Autodesk Fusion 360 part; units mm, degrees
sketch "Boceto1" plane through (0, 0, 0) normal (0, 0, 1) x (1, 0, 0)
  line L0 (0, -31.5) -> (3, -31.5) construction
  circle A0 centre (3, -22.5) radius 1.5 construction
  circle A1 centre (3, -10.5) radius 1.5 construction
  circle A2 centre (-5.5, -17.5) radius 1.5 construction
  line L1 (0, -35) -> (0, -31.5) construction
  line L2 (0, -35) -> (0, -5) construction
  line L3 (0, -20) -> (7.4517, -20) construction
  circle A3 centre (0, -16.5) radius 1.5 construction
  circle A4 centre (5.5, -17.5) radius 1.5 construction
  circle A5 centre (-3, -22.5) radius 1.5 construction
  circle A6 centre (-3, -10.5) radius 1.5 construction
  line L4 (0, -20) -> (-7.4517, -20) construction
  circle A7 centre (-5.5, -26.5) radius 1.5 construction
  line L5 (8.9851, -26.5171) -> (5.0484, -9.7858)
  arc A8 (-8.9851, -26.5171) -> (8.9851, -26.5171) centre (0, -26) ccw
  circle A9 centre (0, -26.5) radius 1.5 construction
  circle A10 centre (5.5, -26.5) radius 1.5 construction
  circle A11 centre (3, -31.5) radius 1.5 construction
  line L6 (0, -26.5) -> (5.5, -26.5) construction
  circle A12 centre (-3, -31.5) radius 1.5 construction
  line L7 (0, -35) -> (0, -26.5) construction
  line L8 (-5.0484, -9.7858) -> (-8.9851, -26.5171)
  arc A13 (5.0484, -9.7858) -> (-5.0484, -9.7858) centre (0, -10.0556) ccw
  arc A14 (6.0413, -9.6396) -> (-6.0413, -9.6396) centre (0, -10.0556) ccw
  line L9 (-6.0413, -9.6396) -> (-9.9909, -26.4257)
  arc A15 (-9.9909, -26.4257) -> (9.9909, -26.4257) centre (0, -26) ccw
  line L10 (9.9909, -26.4257) -> (6.0413, -9.6396)
  line L11 (5.5, -17.5) -> (4.5, -17.5) construction
  line L12 (-5.5, -17.5) -> (-4.5, -17.5) construction
  circle A16 centre (4.5, -17.5) radius 1.5 construction
  circle A17 centre (-4.5, -17.5) radius 1.5 construction
  line L13 (3, -10.5) -> (2.5, -10.5) construction
  line L14 (-3, -10.5) -> (-2.5, -10.5) construction
  circle A18 centre (2.5, -10.5) radius 1.5 construction
  circle A19 centre (-2.5, -10.5) radius 1.5 construction
  dimension "d3" = 0
  dimension "d4" = 9
  dimension "d7" = 0
  dimension "d8" = 10
  dimension "d11" = 0
  dimension "d12" = 21
  dimension "d15" = 0
  dimension "d16" = 9
  dimension "d17" = 3
  dimension "d18" = 3.5
  dimension "d19" = 3
  dimension "d20" = 3
  dimension "d21" = 3
  dimension "d22" = 5
  dimension "d23" = 5.5
  dimension "d24" = 1
  dimension "d48" = 1
  dimension "d49" = 1
  dimension "d50" = 3
  dimension "d51" = 3
  dimension "d52" = 0.5
  dimension "d53" = 3
  dimension "d54" = 3
extrude "Extruir1" add sketch "Boceto1" along normal blind 29
sketch "Boceto2" plane through (0, 0, 29) normal (0, 0, 1) x (-1, 0, 0)
  arc A0 (-5.0484, 9.7858) -> (5.0484, 9.7858) centre (0, 10.0556) ccw
  line L0 (-5.0484, 9.7858) -> (-8.9851, 26.5171)
  arc A1 (8.9851, 26.5171) -> (-8.9851, 26.5171) centre (0, 26) ccw
  line L1 (8.9851, 26.5171) -> (5.0484, 9.7858)
  line L2 (-9.9909, 26.4257) -> (-6.0413, 9.6396)
  arc A2 (-6.0413, 9.6396) -> (6.0413, 9.6396) centre (0, 10.0556) ccw
  line L3 (6.0413, 9.6396) -> (9.9909, 26.4257)
  arc A3 (9.9909, 26.4257) -> (-9.9909, 26.4257) centre (0, 26) ccw
  circle A4 centre (-5.5, 26.5) radius 1.5
  circle A5 centre (-3, 31.5) radius 1.5
  circle A6 centre (3, 31.5) radius 1.5
  circle A7 centre (0, 26.5) radius 1.5
  line L4 (0, 35) -> (0, 26.5)
  circle A8 centre (-3, 22.5) radius 1.5
  circle A9 centre (-5.5, 17.5) radius 1.5
  circle A10 centre (-3, 10.5) radius 1.5
  circle A11 centre (3, 10.5) radius 1.5
  circle A12 centre (0, 16.5) radius 1.5
  circle A13 centre (5.5, 17.5) radius 1.5
  circle A14 centre (3, 22.5) radius 1.5
  circle A15 centre (5.5, 26.5) radius 1.5
  line L5 (-3, 31.5) -> (-5.5, 26.5) construction
  line L6 (3, 31.5) -> (5.5, 26.5) construction
  line L7 (-3, 22.5) -> (0, 26.5) construction
  line L8 (-3, 22.5) -> (-5.5, 26.5) construction
  line L9 (-5.5, 17.5) -> (-3, 22.5) construction
  line L10 (-5.5, 17.5) -> (0, 16.5) construction
  line L11 (0, 16.5) -> (-3, 10.5) construction
  line L12 (-4.25, 29) -> (-7.6694, 30.7097)
  line L13 (-4.25, 24.5) -> (-7.9643, 22.1786)
  line L14 (-4.25, 20) -> (-7.8786, 21.8143)
  line L15 (-3, 28.375) -> (2.011, 25.8695) construction
  line L16 (-3, 25.2812) -> (3.382, 29.27) construction
  line L17 (-3, 26.5) -> (-3, 28.375)
  line L18 (0, 23.6397) -> (-3, 25.3603)
  line L19 (0, 30.75) -> (-3, 28.375)
  line L20 (-4.25, 29) -> (-3, 28.375)
  line L21 (-4.25, 24.5) -> (-2.9341, 25.3225)
  line L22 (-4.25, 20) -> (0, 20)
  line L23 (-1.5, 13.5) -> (0, 13.5)
  line L24 (-1.5, 13.5) -> (-5.5795, 12.043)
  line L25 (0, 30.75) -> (3, 28.375)
  line L26 (4.25, 29) -> (7.6694, 30.7097)
  line L27 (4.25, 29) -> (3, 28.375)
  line L28 (3, 26.5) -> (3, 28.375)
  line L29 (3, 25.3603) -> (3, 25.2812)
  line L30 (0, 23.6397) -> (3, 25.3603)
  line L31 (4.25, 24.5) -> (2.9341, 25.3225)
  line L32 (4.25, 24.5) -> (7.9643, 22.1786)
  line L33 (4.25, 20) -> (7.8786, 21.8143)
  line L34 (4.25, 20) -> (0, 20)
  line L35 (1.5, 13.5) -> (5.5795, 12.043)
  line L36 (1.5, 13.5) -> (0, 13.5)
  line L37 (-1.5866, 14) -> (-5.7476, 12.5139)
  line L38 (-1.5866, 14) -> (0, 14)
  line L39 (-4.368, 19.5) -> (0, 19.5)
  line L40 (-4.368, 19.5) -> (-8.1022, 21.3671)
  line L41 (-3, 26.5) -> (-3, 25.3603)
  line L42 (3, 26.5) -> (3, 25.3603)
  line L43 (0, 30.1123) -> (-2.5, 28.1331)
  line L44 (-2.5, 26.5) -> (-2.5, 28.1331)
  line L45 (-2.5, 26.5) -> (-2.5, 25.6499)
  line L46 (0, 24.2161) -> (-2.5, 25.6499)
  line L47 (0, 24.2161) -> (2.5, 25.6499)
  line L48 (2.5, 26.5) -> (2.5, 25.6499)
  line L49 (2.5, 26.5) -> (2.5, 28.1331)
  line L50 (0, 30.1123) -> (2.5, 28.1331)
  line L51 (-4.515, 24.924) -> (-8.2293, 22.6026)
  line L52 (-4.515, 24.924) -> (-3, 25.8709)
  line L53 (4.515, 24.924) -> (3, 25.8709)
  line L54 (4.515, 24.924) -> (8.2293, 22.6026)
  line L55 (-4.0264, 29.4472) -> (-7.4457, 31.1569)
  line L56 (-4.0264, 29.4472) -> (-2.5672, 28.7176)
  line L57 (3, 28.934) -> (7.4457, 31.1569)
  line L58 (4.0264, 29.4472) -> (2.5672, 28.7176)
  line L59 (2.8037, 19.5) -> (2.7874, 19.5894)
  line L60 (4.368, 19.5) -> (8.1022, 21.3671)
  line L61 (4.368, 19.5) -> (0, 19.5)
  line L62 (1.5866, 14) -> (0, 14)
  line L63 (1.5866, 14) -> (5.7476, 12.5139)
  line L64 (0, 5) -> (0, 13.5)
  line L65 (0.25, 5) -> (0.25, 13.5)
  line L66 (-0.25, 5) -> (-0.25, 13.5)
  line L67 (-0.25, 23.7831) -> (-0.25, 20)
  line L68 (0.25, 23.7831) -> (0.25, 20)
  line L69 (-0.25, 35) -> (-0.25, 30.5521)
  line L70 (0.25, 35) -> (0.25, 30.5521)
  line L71 (0, 26.5) -> (0, 25)
  line L72 (0, 20) -> (0, 19.5)
  line L73 (0, 18) -> (0, 16.5)
  line L74 (-3.2659, 16.9578) -> (-3.2419, 17.0894)
  line L75 (-2.75, 17) -> (-2.75, 19.5)
  line L76 (-2.75, 17) -> (-2.75, 13.5845)
  line L77 (-2.75, 19.5) -> (-2.25, 19.5)
  line L78 (-2.25, 19.5) -> (-2.25, 13.7631)
  line L79 (2.25, 19.5) -> (2.25, 13.7631)
  line L80 (2.75, 17) -> (2.75, 13.5845)
  line L81 (2.75, 17) -> (2.75, 19.5)
  dimension "d27" = 7
  dimension "d28" = 9
  dimension "d29" = -0.5
  dimension "d31" = 0.5
  dimension "d32" = -0.5
  dimension "d38" = 0.5
  dimension "d39" = -0.5
  dimension "d40" = 0.25
  dimension "d41" = -0.25
  dimension "d55" = 0.5
extrude "Extruir2" add sketch "Boceto2" against normal blind 23.5 contours A0 L23 L64 L66 | L0 L1 L23 L24 L35 L36 L37 L38 L62 L63 | A0 L36 L64 L65 | L37 L39 L75 L76 L77 L78 | L0 L14 L22 L39 L40 L72 L77 | L1 L33 L34 L60 L61 L72 | L61 L63 L79 L80 L81 | L0 L13 L18 L21 L41 L51 L52 | L18 L22 L30 L34 L67 L68 | L17 L18 L19 L25 L28 L30 L41 L42 | A1 L12 L19 L20 L55 L56 | L1 L29 L31 L32 L42 L53 L54 | A1 L4 L19 L69 | A1 L4 L25 L70 | A1 L25 L26 L27 L57 L58
equation "d25 = 5 mm + 18 mm + 5 mm + 1 mm"
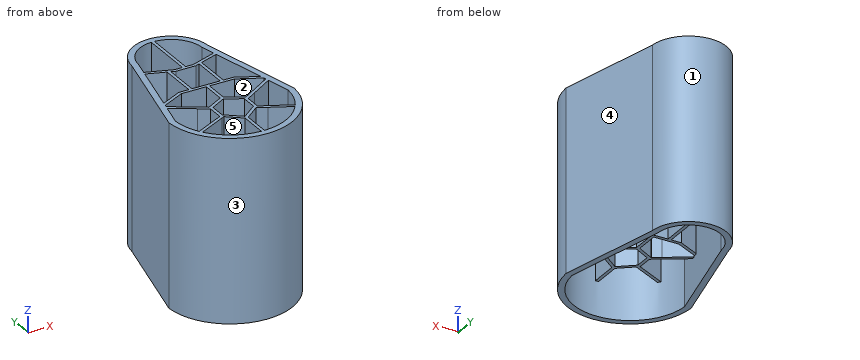
Verification items for the finished model (mm, model axes). Face numbers are marked on the shaded views. A direction names the side the tool comes from. Give positions to 0.01 mm unless a question says otherwise; leave off trailing zeros. Order: outer loops, then holes, each group sorted by start corner. A loop starts at its lowest first (then second) coordinate and runs counter-clockwise, first axis right, second up. Notation, with made-up numbers: M 50.25,29 L 60.25,29 A15 cw 60.25,55 Z; hole C -39,-12 d10. An arc over 180 degrees is marked long. Answer in a Markdown table with one row per item. Add a question column.
Item 1: Tool access check on the marked faces 1 and 2. Record the directions out of +Z, -Z, +X, -X, +Y, -Y that give a thin tool (end or side, any length) a straight path to the whole face; none if there is none.
Item 2: Mould release check, pull along X, two halves, no side actions. Record for the marked faces 3, 4 and 5: released by +X, released by -X, zero draft, split by the parting line, or undercut.
Item 3: Section check C-C, the plane z = 20.75. State how many separate pieces and enclosed holes the cut face has, and give its area (3 significant figures).
Item 4: Section check A-A, the plane x = 8.5. Enter the section's corners in (y, z), and give its area (3 significant figures).
Item 5: Gauge pin test, flat ends, axial feed: pin 1 (5 mm diameter, centred on x = -0.5, z = 13.5, fed in from -Y); pin 2 (3 mm diameter, centred on y = -22, z = 18, fed in from +X); pin 3 (4 mm diameter, centred on x = -7, z = 19, fed in from +Y); pin 4 (1.8 mm diameter, centred on x = -4, z = 23, fed in from +Y). Record the tip position at first contact, or that the pin passes through.
Item 6: Section check B-B, the plane y = -8. Enter the section's corners in (x, z), and give its area (3 significant figures).
Item 7: Scan lines: probe 1 along X at (y, z) = (-18, 11); probe 2 along X at (y, z) = (-8.5, 20.75); probe 3 along Y at (x, z) = (-1, 18.5). Record each from-to range of solid material in increasing order. Write a range as from..to.
Filled sheet:
| question | item | result |
|---|---|---|
| 1 | face 1 | +Z, -Z, +Y |
| 1 | face 2 | +Z, -Z |
| 2 | face 3 | split by the parting line |
| 2 | face 4 | released by +X |
| 2 | face 5 | undercut |
| 3 | separate pieces | 1 |
| 3 | enclosed holes | 12 |
| 3 | area | 129 mm^2 |
| 4 | outline | M -31.27,0 L -28.96,0 L -28.96,29 L -31.27,29 Z; M -24.46,0 L -20.09,0 L -20.09,29 L -24.46,29 Z |
| 4 | area | 194 mm^2 |
| 5 | pin 1 | stops at y = -36 |
| 5 | pin 2 | stops at x = 9.3 |
| 5 | pin 3 | stops at y = -6.64 |
| 5 | pin 4 | stops at y = -4.85 |
| 6 | outline | M -5.7,0 L -4.62,0 L -4.62,29 L -5.7,29 Z; M -0.25,5.5 L 0.25,5.5 L 0.25,29 L -0.25,29 Z; M 4.62,0 L 5.7,0 L 5.7,29 L 4.62,29 Z |
| 6 | area | 74.2 mm^2 |
| 7 | probe 1 | x = -8.01..-6.98, -2.75..-2.25, 2.25..2.75, 6.98..8.01 |
| 7 | probe 2 | x = -5.85..-4.81, -0.25..0.25, 4.81..5.85 |
| 7 | probe 3 | y = -35.95..-34.94, -29.96..-29.32, -24.79..-24.21, -20..-19.5, -14..-13.5, -5.1..-4.08 |
